```python
from build123d import *

# Parameters (mm, degrees)
ESQUISSE1_W               = 75
ESQUISSE1_H               = 105
BOSS_EXTRU_1_DEPTH        = 1
ENL_V_MAT_EXTRU_1_REACH   = 66.525
ESQUISSE3_R               = 2
SYM_TRIE2_COPY_1_REACH    = 66.525
SYM_TRIE2_COPY_1_SKETCH_R = 2
ESQUISSE5_W               = 9
ESQUISSE5_H               = 11
BOSS_EXTRU_3_DEPTH        = 10
ESQUISSE5_2_W             = 9
ESQUISSE5_2_H             = 11
BOSS_EXTRU_4_DEPTH        = 4
ESQUISSE6_W               = 8.451892611
ESQUISSE6_H               = 13.39545244
BOSS_EXTRU_5_DEPTH        = 15


with BuildPart() as part:
    # Esquisse1 → Boss.-Extru.1 (new body)
    with BuildSketch(Plane.XY):
        Rectangle(ESQUISSE1_W, ESQUISSE1_H)
    extrude(amount=BOSS_EXTRU_1_DEPTH)

    # Esquisse3 → Enlèv. mat.-Extru.1 (cut, up to next)
    with BuildSketch(Plane.XY.offset(1), mode=Mode.PRIVATE) as enl_v_mat_extru_1_sk1:
        with Locations((-33, -48)):
            Circle(ESQUISSE3_R)
    enl_v_mat_extru_1_tool1 = extrude(enl_v_mat_extru_1_sk1.sketch, amount=-ENL_V_MAT_EXTRU_1_REACH, mode=Mode.PRIVATE) & part.part
    enl_v_mat_extru_1 = enl_v_mat_extru_1_tool1.solids().sort_by_distance((-33, -48, 1))[0]
    add(enl_v_mat_extru_1, mode=Mode.SUBTRACT)

    # Symétrie1: Enlèv. mat.-Extru.1 across plane
    add(enl_v_mat_extru_1.mirror(Plane(origin=(0, 0, 0), x_dir=(0, 0, 1), z_dir=(1, 0, 0))), mode=Mode.SUBTRACT)

    # Symétrie2: Enlèv. mat.-Extru.1 across plane
    add(enl_v_mat_extru_1.mirror(Plane.ZX), mode=Mode.SUBTRACT)

    # Symétrie2 copy 1 sketch → Symétrie2 copy 1 (cut, up to next)
    with BuildSketch(Plane(origin=(0, 0, 1), x_dir=(-1, 0, 0), z_dir=(0, 0, 1)), mode=Mode.PRIVATE) as sym_trie2_copy_1_sk1:
        with Locations((-33, -48)):
            Circle(SYM_TRIE2_COPY_1_SKETCH_R)
    sym_trie2_copy_1_tool1 = extrude(sym_trie2_copy_1_sk1.sketch, amount=-SYM_TRIE2_COPY_1_REACH, mode=Mode.PRIVATE) & part.part
    add(sym_trie2_copy_1_tool1.solids().sort_by_distance((33, 48, 1))[0], mode=Mode.SUBTRACT)

    # Esquisse5 → Boss.-Extru.3 (add)
    with BuildSketch(Plane.XZ.offset(52.5)):
        with Locations((25, 6.5)):
            Rectangle(ESQUISSE5_W, ESQUISSE5_H)
    extrude(amount=-BOSS_EXTRU_3_DEPTH)

    # Esquisse5<2> → Boss.-Extru.4 (add)
    with BuildSketch(Plane.XZ.offset(52.5)):
        with Locations((25, 6.5)):
            Rectangle(ESQUISSE5_2_W, ESQUISSE5_2_H)
    extrude(amount=BOSS_EXTRU_4_DEPTH)

    # Esquisse6 → Boss.-Extru.5 (add)
    with BuildSketch(Plane.XY.offset(1)):
        with Locations((31.335790529, -33.335790529)):
            Rectangle(ESQUISSE6_W, ESQUISSE6_H)
    extrude(amount=BOSS_EXTRU_5_DEPTH)


solid = part.part
```
Could you check a few things on this model? Use its own coordinates, in mm. A direction names the side the tool comes from. Coordinates: 2 decimals unless noted, no trailing zeros. Order: outer loops, then holes, each group sorted by start corner. A loop starts at its lowest first (then second) coordinate and runs counter-clockwise, first axis right, second up. Notation, with made-up numbers: M 84,-2.75 L 124,-2.75 A18 cw 124,4.25 Z; hole C 22.25,28.25 d6. An arc over 180 degrees is marked long. Use a Markdown table: item, result. Add a question column.
Q1. I want a section at B-B on y = 48. List the corners of the cut face in (x, z) for me.
Q2. I'm going to push flat-ended pins straight in: pin 1 (7 mm diameter, centred on x = 23, y = -46.5, fed in from +Z); pin 2 (4 mm diameter, centred on y = -27.5, z = 12, fed in from +X); pin 3 (4.5 mm diameter, centred on x = -33, y = 48, fed in from +Z). Where does each tip first touch, or does it pass through?
Q3. I want a section at D-D on y = -48. List the corners of the cut face in (x, z) for me.
Q4. Which directions (+Z, -Z, +X, -X, +Y, -Y) give clear straight access to the entire face, cutting with the end or side of a thin tool? Please do faces 1 (the flat face through (25, -49, 12)), 2 (the flat face through (20.5, -49, 6)), 3 (the flat face through (25, -42.5, 7)), 4 (the flat face through (29.5, -49, 6)).
Q5. I want a section at C-C on x = -33. List the corners of the cut face in (y, z) for me.
Q6. If I drill on L1, parallel to X at y = 48, z = 0.3; L2, parallel to Y at x = -33, z = 0.3; L3, parallel to Y at x = -5, z = 0.75, over which ranges is the centre line in solid material (lowest first)?
Q7. We'd pull the mould along X, two halves only. Please class faces 5 (the flat face through (25, -54, 1)), 6 (the flat face through (27.11, -33, 8)), 7 (the cylindrical face through (32.077, -49.774, 0.507)): pulls with the +X half, pulls with the -X half, needs draft (parallel to the pull), parting line crosses it, or undercut.
Q8. I want a section at A-A on z = 3.5. List the corners of the cut face in (x, y) for me, then the cut area to 3 significant figures.
Checked values:
| question | item | result |
|---|---|---|
| 1 | outline | M -37.5,0 L -35,0 L -35,1 L -37.5,1 Z; M -31,0 L 31,0 L 31,1 L -31,1 Z; M 35,0 L 37.5,0 L 37.5,1 L 35,1 Z |
| 2 | pin 1 | z = 12 |
| 2 | pin 2 | x = 35.56 |
| 2 | pin 3 | z = 1 |
| 3 | outline | M -37.5,0 L -35,0 L -35,1 L -37.5,1 Z; M -31,0 L 31,0 L 31,1 L 29.5,1 L 29.5,12 L 20.5,12 L 20.5,1 L -31,1 Z; M 35,0 L 37.5,0 L 37.5,1 L 35,1 Z |
| 4 | face 1 | +Z, +X, -X, -Y |
| 4 | face 2 | +Z, -X, +Y, -Y |
| 4 | face 3 | +Z, +X, -X |
| 4 | face 4 | +Z, +X, -Y |
| 5 | outline | M -52.5,0 L -50,0 L -50,1 L -52.5,1 Z; M -46,0 L 46,0 L 46,1 L -46,1 Z; M 50,0 L 52.5,0 L 52.5,1 L 50,1 Z |
| 6 | L1 | -37.5 to -35, -31 to 31, 35 to 37.5 |
| 6 | L2 | -52.5 to -50, -46 to 46, 50 to 52.5 |
| 6 | L3 | -52.5 to 52.5 |
| 7 | face 5 | needs draft |
| 7 | face 6 | pulls with the -X half |
| 7 | face 7 | undercut |
| 8 | outline | M 20.5,-56.5 L 29.5,-56.5 L 29.5,-42.5 L 20.5,-42.5 Z; M 27.11,-40.03 L 35.56,-40.03 L 35.56,-26.64 L 27.11,-26.64 Z |
| 8 | area | 239 mm² |
